Here's how the part is built. I have some questions about the finished solid (model axes, mm). A direction names the side the tool comes from. Coordinates: 2 decimals unless noted, no trailing zeros. Order: outer loops, then holes, each group sorted by start corner. A loop starts at its lowest first (then second) coordinate and runs counter-clockwise, first axis right, second up. Notation, with made-up numbers: (-11, 19) - (21, 19) arc R21 cw to (21, 27) - close; hole circle Ø1 at (80.25, -38). An arc over 180 degrees is marked (long way). Use one line per item in the form item = value. Start each with the question number.
from build123d import *

# Parameters (mm, degrees)
BOSS_EXTRUDE1_DEPTH = 72
SKETCH2_W           = 10
SKETCH2_H           = 36
CUT_EXTRUDE1_DEPTH  = 72
SKETCH3_R           = 12
CUT_EXTRUDE3_DEPTH  = 12
CUT_EXTRUDE4_DEPTH  = 32
SKETCH5_W           = 70.022826976
SKETCH5_H           = 12
BOSS_EXTRUDE2_DEPTH = 5


with BuildPart() as part:
    # Sketch1 → Boss-Extrude1 (new body)
    with BuildSketch(Plane.XY):
        Polygon((0, 0), (70, 1.787819253), (70, -3.212180747), (145, -1.296660118), (145, 23.703339882), (35, 20.893909627), (35, 90), (0, 90), align=None)
    extrude(amount=-BOSS_EXTRUDE1_DEPTH)

    # Sketch2 → Cut-Extrude1 (cut)
    with BuildSketch(Plane.XY):
        with Locations((5, 48)):
            Rectangle(SKETCH2_W, SKETCH2_H)
    extrude(amount=-CUT_EXTRUDE1_DEPTH, mode=Mode.SUBTRACT)

    # Sketch3 → Cut-Extrude3 (cut)
    with BuildSketch(Plane(origin=(0, 0, 0), x_dir=(0, 0, -1), z_dir=(1, 0, 0))):
        with Locations(Location((35.804414242, 47.892382062, 0), (0, 0, 90))):
            Circle(SKETCH3_R)
        with BuildLine():
            Line((59.723322508, 66), (11.885505976, 66))
            ThreePointArc((11.885505976, 66), (35.804414242, 77.892382062), (59.723322508, 66))
        make_face()
        with BuildLine():
            Line((59.88475195, 30), (11.724076534, 30))
            ThreePointArc((11.724076534, 30), (35.804414242, 17.892382062), (59.88475195, 30))
        make_face()
    extrude(amount=CUT_EXTRUDE3_DEPTH, mode=Mode.SUBTRACT)

    # Sketch4 → Cut-Extrude4 (cut)
    with BuildSketch(Plane(origin=(-0.510472517, 19.986962392, 0), x_dir=(0.9996740066520181, 0.025531949089344263, 0), z_dir=(-0.025531949089344263, 0.9996740066520181, 0))):
        with BuildLine():
            Line((99.920378063, 47.920353232), (145.536976224, 47.999981717))
            ThreePointArc((145.536976224, 47.999981717), (157.557905149, 36.020947208), (145.57887064, 24.000018283))
            Line((145.57887064, 24.000018283), (99.962272479, 23.920389797))
            ThreePointArc((99.962272479, 23.920389797), (87.941343554, 35.899424307), (99.920378063, 47.920353232))
        make_face()
    extrude(amount=-CUT_EXTRUDE4_DEPTH, mode=Mode.SUBTRACT)

    # Sketch5 → Boss-Extrude2 (add)
    with BuildSketch(Plane(origin=(0, 0, 0), x_dir=(0.9996740066520181, 0.025531949089344187, 0), z_dir=(0.025531949089344187, -0.9996740066520181, 0))):
        with Locations((35.011413488, -66)):
            Rectangle(SKETCH5_W, SKETCH5_H)
    extrude(amount=BOSS_EXTRUDE2_DEPTH)


solid = part.part
1) Suppose I cut it at A-A, the plane x = 125. List the corners of the cut face in (y, z) for me.
2) For pin 1 (5 mm diameter, centred on y = 46, z = -36.5, fed in from +X); pin 2 (6 mm diameter, centred on x = 88, z = -37.5, fed in from -Y); pin 3 (5.5 mm diameter, centred on x = 46.5, y = -2.5, fed in from +Z), each with a flat end and sliding along its axis, tell me the tip position at first contact or that it passes through.
3) If we mould it in two halves opening along Z, with no side actions, what happens to faces 1 (the flat face through (5, 66, -6)), 2 (the flat face through (34, 33, -72)), 3 (the flat face through (12, 71, -36))? For each: pulls with the +Z half, pulls with the -Z half, needs draft (parallel to the pull), parting line crosses it, or undercut.
4) I need wall thicknesses on probe 1 along Z at (x, y) = (106.5, 16); probe 2 along X at (y, z) = (39.5, -56); probe 3 along X at (y, z) = (78.5, -35). Which ranges of each line are inside material? Lowest first, please. Write a range as [from, to].
5) Which directions (+Z, -Z, +X, -X, +Y, -Y) give clear straight access to the entire face, cutting with the end or side of a thin tool? Please do faces 4 (the flat face through (5, 30, -66)), 5 (the flat face through (35, -2, -60)), 6 (the cylindrical face through (5.92, 77.89, -35.42)).
6) Suppose I cut it at C-C, the plane y = 49. List the corners of the cut face in (x, z) for me.
7) Suppose I cut it at B-B, the plane z = -51. List the corners of the cut face in (x, y) for me.
8) Suppose I cut it at D-D, the plane x = 54. List the corners of the cut face in (y, z) for me, then the cut area to 3 significant figures.
From the geometry:
q1.outline = (-1.81, -72) - (23.19, -72) - (23.19, -47.97) - (-1.81, -47.96) - close; (-1.81, -23.96) - (23.19, -23.97) - (23.19, 0) - (-1.81, 0) - close
q2.pin_1 = 35
q2.pin_2 = -2.83
q2.pin_3 = -60
q3.face_1 = needs draft
q3.face_2 = pulls with the -Z half
q3.face_3 = undercut
q4.probe_1 = [-72, -47.93], [-23.93, 0]
q4.probe_2 = [10, 35]
q4.probe_3 = [0, 35]
q5.face_4 = +Z, -Z, -X
q5.face_5 = +Z, -Y
q5.face_6 = -X
q6.outline = (10, -72) - (35, -72) - (35, 0) - (10, 0) - (10, -23.86) - (12, -23.86) - (12, -47.75) - (10, -47.75) - close
q7.outline = (0, 0) - (70, 1.79) - (70, -3.21) - (145, -1.3) - (145, 23.7) - (35, 20.89) - (35, 90) - (0, 90) - (0, 73.76) - (12, 73.76) - (12, 66) - (10, 66) - (10, 30) - (12, 30) - (12, 22.03) - (0, 22.03) - close
q8.outline = (-3.62, -72) - (21.38, -72) - (21.38, 0) - (1.38, 0) - (1.38, -60) - (-3.62, -60) - close
q8.area = 1,500 mm2
